```python
from build123d import *

# Parameters (mm, degrees)
SKETCH2_W           = 30
SKETCH2_H           = 15
SKETCH2_W_2         = 26
SKETCH2_H_2         = 9.2
BOSS_EXTRUDE1_DEPTH = 150
BOSS_EXTRUDE2_DEPTH = 5
FILLET1_R           = 3
LPATTERN1_COUNT     = 15
LPATTERN1_PITCH     = 10


with BuildPart() as part:
    # Sketch2 → Boss-Extrude1 (new body)
    with BuildSketch(Plane(origin=(0, 0, 0), x_dir=(1, 0, 0), z_dir=(0, 1, 0))):
        Rectangle(SKETCH2_W, SKETCH2_H)
        with Locations((0, -1.1)):
            Rectangle(SKETCH2_W_2, SKETCH2_H_2, mode=Mode.SUBTRACT)
    extrude(amount=BOSS_EXTRUDE1_DEPTH)

    # Sketch3 → Boss-Extrude2 (add)
    with BuildSketch(Plane(origin=(0, 150, 0), x_dir=(1, 0, 0), z_dir=(0, 1, 0))):
        Polygon((-2.87163554, -5.7), (-2.87163554, -3.7), (3.631457211, -3.7), (3.631457211, -5.7), (5.631457211, -5.7), (5.631457211, -1.7), (-4.87163554, -1.7), (-4.87163554, -5.7), align=None)
    boss_extrude2 = extrude(amount=-BOSS_EXTRUDE2_DEPTH)

    # Fillet1
    fillet1_edges = [part.edges().sort_by_distance(p)[0] for p in [
        (-13, 75, -3.5),
        (-13, 75, 5.7),
        (13, 75, 5.7),
        (13, 75, -3.5),
        (-15, 75, -7.5),
        (15, 75, -7.5),
        (15, 75, 7.5),
        (-15, 75, 7.5),
    ]]
    fillet(fillet1_edges, radius=FILLET1_R)

    # LPattern1: Boss-Extrude2 ×15
    with Locations(*[(0, -i * LPATTERN1_PITCH, 0) for i in range(1, LPATTERN1_COUNT)]):
        add(boss_extrude2)


solid = part.part
```
Geometry: final body of the model. Coordinates: model frame, mm. A direction names the side the tool comes from. Round coordinates to 2 decimals unless told otherwise and drop trailing zeros. Order: outer loops, then holes, each group sorted by start corner. A loop starts at its lowest first (then second) coordinate and runs counter-clockwise, first axis right, second up. Notation, with made-up numbers: M 68,1 L 80,1 A30 cw 80,39 Z; hole C -15.5,76 d9. An arc over 180 degrees is marked long. One line per item, written item: value.
(1) Cut plane A-A (y = 128). Return the cut outline in (x, z).
Result sheet:
outline: M -15,-4.5 A3 ccw -12,-7.5 L 12,-7.5 A3 ccw 15,-4.5 L 15,4.5 A3 ccw 12,7.5 L -12,7.5 A3 ccw -15,4.5 Z; hole M -13,-0.5 A3 ccw -10,-3.5 L 10,-3.5 A3 ccw 13,-0.5 L 13,2.7 A3 ccw 10,5.7 L 5.63,5.7 L 5.63,1.7 L -4.87,1.7 L -4.87,5.7 L -10,5.7 A3 ccw -13,2.7 Z; hole M -2.87,3.7 L 3.63,3.7 L 3.63,5.7 L -2.87,5.7 Z
(2) Cut plane D-D (z = -1.75). Return the cut outline in (x, y).
Result sheet:
outline: M -15,0 L -12.73,0 L -12.73,150 L -15,150 Z; M 12.73,0 L 15,0 L 15,150 L 12.73,150 Z
(3) Pull-direction query (Y, two-part tool) for faces 1 (the flat face through (0, 74, 7.5)), 2 (the flat face through (0, 30, 3)); classes: pulls with the +Y half, pulls with the -Y half, needs draft (parallel to the pull), parting line crosses it, or undercut.
Result sheet:
face 1: needs draft
face 2: undercut
(4) Cut plane B-B (x = -8). Return the cut outline in (y, z), and give its area (3 significant figures).
Result sheet:
outline: M 0,-7.5 L 150,-7.5 L 150,-3.5 L 0,-3.5 Z; M 0,5.7 L 150,5.7 L 150,7.5 L 0,7.5 Z
area: 870 mm2
(5) Line query: probe 1 along Z at (x, y) = (6.75, 82); probe 2 along X at (y, z) = (104, 2.5); probe 3 along X at (y, z) = (39.5, -3). Output: solid intervals per line, ascending. Write a range as [from, to].
Result sheet:
probe 1: [-7.5, -3.5], [5.7, 7.5]
probe 2: [-15, -13], [13, 15]
probe 3: [-15, -11.66], [11.66, 15]
(6) Cut plane C-C (y = 53). Return the cut outline in (x, z).
Result sheet:
outline: M -15,-4.5 A3 ccw -12,-7.5 L 12,-7.5 A3 ccw 15,-4.5 L 15,4.5 A3 ccw 12,7.5 L -12,7.5 A3 ccw -15,4.5 Z; hole M -13,-0.5 A3 ccw -10,-3.5 L 10,-3.5 A3 ccw 13,-0.5 L 13,2.7 A3 ccw 10,5.7 L -10,5.7 A3 ccw -13,2.7 Z
(7) Reachability of faces 3 (the flat face through (0, 70, 3)), 4 (the flat face through (15, 74, 0)), 5 (the flat face through (5.631, 138, 4)) from +Z, -Z, +X, -X, +Y, -Y: full face, straight path, thin tool, end or side. Return the list, or none.
Result sheet:
face 3: none
face 4: +Z, -Z, +X, +Y, -Y
face 5: +Y, -Y
(8) Pin query (flat end, axial travel): P1, Ø1.5, axis at y = 62, z = 5, coming from the -X side; P2, Ø0.6, axis at y = 6.5, z = 5, coming from the +X side; P3, Ø1.2, axis at x = -0.5, z = 3, coming from the -Y side; P4, Ø1.2, axis at x = -1.5, z = 4.5, coming from the +Y side. Return the tip coordinate at first contact, or that it passes through.
Result sheet:
P1: x = -15
P2: x = 14.99
P3: y = 5
P4: through
